Autodesk Inventor part; units mm, degrees
ref_plane "YZ Plane" through (0, 0, 0) normal (1, 0, 0) x (0, 1, 0)
ref_plane "XZ Plane" through (0, 0, 0) normal (0, 1, 0) x (-1, 0, 0)
ref_plane "XY Plane" through (0, 0, 0) normal (0, 0, 1) x (1, 0, 0)
sketch "Skizze1" plane through (0, 0, 0) normal (0, 1, 0) x (-1, 0, 0)
  circle A0 centre (0, 0) radius 81
  dimension "d0" = 162
extrude "Extrusion1" add sketch "Skizze1" along normal blind 5
sketch "Skizze2" plane through (0, 5, 0) normal (0, 1, 0) x (1, 0, 0)
  circle A0 centre (0, 0) radius 70
  circle A1 centre (0, 0) radius 20
  circle A2 centre (0, 0) radius 81
  circle A3 centre (0, 0) radius 76
  point P0 (-17.3365, 0)
  point P1 (-14.3955, 0)
  point P2 (-11.4544, 0)
  point P3 (-8.823, 0)
  point P4 (-5.882, 0)
  point P5 (5.7272, 0)
  point P6 (8.2039, 0)
  point P7 (10.3709, 0)
  point P8 (12.6928, 0)
  point P9 (14.8598, 0)
  point P10 (17.4912, 0)
  dimension "d3" = 140
  dimension "d4" = 40
  dimension "d21" = 152
hole "Bohrung1" at (0, 5, 0) direction (0, -1, 0) diameter 5 end through all
extrude "Extrusion2" add sketch "Skizze2" along normal blind 2.5 contours A2 | A3
hole "Bohrung2" at (-17.3365, 5, 0) at (-14.3955, 5, 0) at (-11.4544, 5, 0) at (-8.823, 5, 0) at (-5.882, 5, 0) at (5.7272, 5, 0) at (8.2039, 5, 0) at (10.3709, 5, 0) at (12.6928, 5, 0) at (14.8598, 5, 0) at (17.4912, 5, 0) direction (0, -1, 0) diameter 0.7 end through all
extrude "Extrusion3" add sketch "Skizze2" along normal blind 33 contours A2
sketch "Skizze3" plane through (0, 38, 0) normal (0, 1, 0) x (1, 0, 0)
  circle A0 centre (39.25, 67.983) radius 1.2
  circle A1 centre (-39.25, 67.983) radius 1.2
  circle A2 centre (39.25, -67.983) radius 1.2
  circle A3 centre (-39.25, -67.983) radius 1.2
  circle A4 centre (78.5, 0) radius 1.2
  circle A5 centre (-78.5, 0) radius 1.2
  point P0 (0, 0)
hole "Bohrung3" at (39.25, 38, -67.983) at (39.25, 38, 67.983) at (-39.25, 38, 67.983) at (-78.5, 38, 0) at (-39.25, 38, -67.983) at (78.5, 38, 0) direction (0, -1, 0) diameter 0.9294 depth 10 tip angle 118
CAD build for the part. Positions are in the model's coordinates, mm. A direction names the side the tool comes from. Round coordinates to 2 decimals unless told otherwise and drop trailing zeros. Write each loop counter-clockwise with the first axis right and the second up, starting at its lowest first coordinate (ties: lowest second). Pieces come first, ordered by that corner, then holes. Notation, with made-up numbers: (35, 39) -> (70, 39) arc R33 ccw to (70, 77) -> close; hole circle Ø11 at (69, 85). An arc over 180 degrees is marked (long way). Answer in a Markdown table with one row per item. Add a question column.
Item 1: Drill centre lines: line 1 (X direction, y = 34.25, z = 0); line 2 (X direction, y = 35, z = -2.5); line 3 (Y direction, x = -45.5, z = -45.5). Where is each one in solid material? Low to high. Write a range as from..to.
Item 2: Which spindle directions (+Z, -Z, +X, -X, +Y, -Y) get a long thin tool onto all of the face, cutting with end or side? Do faces 1 (the face through (60, 38, 48)), 2 (the face through (-55.55, 6.232, -42.594)). Say none if no direction does.
Item 3: Saw through at C-C, the plane z = -27. Write the cut outline in (x, y).
Item 4: Mould opens along Z. For faces 3 (the face through (1, 0, -17)), 4 (the face through (2.44, 2.46, -0.54)), 5 (the face through (5.34, 18.734, 80.824)) say: pulls with the +Z half, pulls with the -Z half, needs draft (parallel to the pull), parting line crosses it, or undercut.
Item 5: Saw through at B-B, the plane y = 25. Write the cut outline in (x, z), then the cut area to 3 significant figures.
Item 6: Drop flat-ended pins along their axis: pin 1 Ø1 at (x, z) = (-37.5, 17) entering from +Y; pin 2 Ø5 at (x, z) = (-55.5, 47.5) entering from +Y; pin 3 Ø3 at (x, z) = (0, 0) entering from +Y; pin 4 Ø5 at (y, z) = (11.5, -20) entering from -X. Give the stop position or say it passes through.
Findings below:
| question | item | result |
|---|---|---|
| 1 | line 1 | x = -81..-78.96, -78.04..-76, 76..78.04, 78.96..81 |
| 1 | line 2 | x = -80.96..-75.96, 75.96..80.96 |
| 1 | line 3 | y = 0..5 |
| 2 | face 1 | +Z, -Z, +X, -X, +Y |
| 2 | face 2 | +Y |
| 3 | outline | (-76.37, 0) -> (76.37, 0) -> (76.37, 38) -> (71.04, 38) -> (71.04, 7.5) -> (64.58, 7.5) -> (64.58, 5) -> (-64.58, 5) -> (-64.58, 7.5) -> (-71.04, 7.5) -> (-71.04, 38) -> (-76.37, 38) -> close |
| 4 | face 3 | needs draft |
| 4 | face 4 | undercut |
| 4 | face 5 | parting line crosses it |
| 5 | outline | circle Ø162 at (0, 0); hole circle Ø152 at (0, 0) |
| 5 | area | 2,470 mm^2 |
| 6 | pin 1 | stops at y = 5 |
| 6 | pin 2 | stops at y = 7.5 |
| 6 | pin 3 | passes through |
| 6 | pin 4 | stops at x = -79.09 |
